Could you check a few things on this model? Use its own coordinates, in mm. A direction names the side the tool comes from. Coordinates: 2 decimals unless noted, no trailing zeros. Order: outer loops, then holes, each group sorted by start corner. A loop starts at its lowest first (then second) coordinate and runs counter-clockwise, first axis right, second up. Notation, with made-up numbers: (-5.75, 28) -> (36.25, 28) arc R16 ccw to (36.25, 42) -> close; hole circle Ø11 at (18.5, 37). An arc over 180 degrees is marked (long way). Use a Markdown table: item, result. Add a question column.
1) If I drill on L1, parallel to Z at x = 1, y = 1; L2, parallel to Z at x = 5, y = 9; L3, parallel to X at y = -0.5, z = -27.5, over which ranges is the centre line in solid material (lowest first)? Write a range as [from, to].
2) Thinking about a two-plate mould opening in X: for faces 1 (the cylindrical face through (-23.31, -13.36, 4.83)), 2 (the flat face through (-15, -3, -3)), 3 (the cylindrical face through (-12.517, -3.694, -1.479)), 4 (the flat face through (12.65, 6.96, 1.48)), which applies, +X half, -X half, draft (parallel to the pull), parting line (faces both ways), or undercut?
3) If we section it at A-A (x = 0): Write out the boundary of the cut face in (y, z), plus the area to 3 significant figures.
4) If we section it at D-D (x = -15): Write out the boundary of the cut face in (y, z), plus the area to 4 significant figures.
5) Will these pins go through, and if not, where does the flat tip stop? pin 1 Ø6 at (x, y) = (17.5, -6) entering from +Z; pin 2 Ø2 at (y, z) = (1, -11) entering from -X; pin 3 Ø1.5 at (x, y) = (-14.5, -3) entering from -Z.
6) If we section it at B-B (z = -27): Write out the boundary of the cut face in (x, y).
7) If we section it at C-C (y = 7): Write out the boundary of the cut face in (x, z), plus the area to 3 significant figures.
8) Which directions (+Z, -Z, +X, -X, +Y, -Y) give clear straight access to the entire face, cutting with the end or side of a thin tool? Please do faces 5 (the flat face through (5, 2, 0)), 6 (the flat face through (-22, -12, 8)), 7 (the flat face through (5, 14, -3)).
```python
from build123d import *

# Parameters (mm, degrees)
BOSS_EXTRUDE1_DEPTH = 3
SKETCH2_R           = 3.5
BOSS_EXTRUDE2_DEPTH = 10
SKETCH3_R           = 2
BOSS_EXTRUDE3_DEPTH = 5
SKETCH4_R           = 2.5
BOSS_EXTRUDE4_DEPTH = 3
CIRPATTERN1_COUNT   = 3
SKETCH5_R           = 3.5
BOSS_EXTRUDE6_DEPTH = 110


with BuildPart() as part:
    # Sketch1 → Boss-Extrude1 (new body)
    with BuildSketch(Plane.XY):
        with BuildLine():
            Line((23.267949192, -11.43375673), (1.732050808, 25.867513459))
            ThreePointArc((1.732050808, 25.867513459), (0, 26.867513459), (-1.732050808, 25.867513459))
            Line((-1.732050808, 25.867513459), (-23.267949192, -11.43375673))
            ThreePointArc((-23.267949192, -11.43375673), (-23.267949192, -13.43375673), (-21.535898385, -14.43375673))
            Line((-21.535898385, -14.43375673), (21.535898385, -14.43375673))
            ThreePointArc((21.535898385, -14.43375673), (23.267949192, -13.43375673), (23.267949192, -11.43375673))
        make_face()
    extrude(amount=BOSS_EXTRUDE1_DEPTH)

    # Sketch2 → Boss-Extrude2 (add)
    with BuildSketch(Plane(origin=(0, 0, 0), x_dir=(-1, 0, 0), z_dir=(0, 0, -1))):
        with Locations(Location((0, 0, 0), (0, 0, 180))):
            Circle(SKETCH2_R)
    extrude(amount=BOSS_EXTRUDE2_DEPTH)

    # Sketch3 → Boss-Extrude3 (add)
    with BuildSketch(Plane.XY.offset(3)):
        with Locations(Location((0, 24.867513459, 0), (0, 0, 150))):
            Circle(SKETCH3_R)
        with Locations(Location((21.535898385, -12.43375673, 0), (0, 0, 270))):
            Circle(SKETCH3_R)
        with Locations(Location((-21.535898385, -12.43375673, 0), (0, 0, 150))):
            Circle(SKETCH3_R)
    extrude(amount=BOSS_EXTRUDE3_DEPTH)

    # Sketch4 → Boss-Extrude4 (add)
    with BuildSketch(Plane(origin=(0, 0, 0), x_dir=(-1, 0, 0), z_dir=(0, 0, -1))):
        with Locations(Location((-10, -11.43375673, 0), (0, 0, 180))):
            Circle(SKETCH4_R)
    boss_extrude4 = extrude(amount=BOSS_EXTRUDE4_DEPTH)

    # CirPattern1: Boss-Extrude4 ×3 about axis
    cirpattern1_axis = Axis((0, 0, 0), (0, 0, 1))
    for i in range(1, CIRPATTERN1_COUNT):
        add(boss_extrude4.rotate(cirpattern1_axis, i * 360 / CIRPATTERN1_COUNT))

    # Sketch5 → Boss-Extrude6 (add)
    with BuildSketch(Plane(origin=(0, 0, -10), x_dir=(-1, 0, 0), z_dir=(0, 0, -1))):
        with Locations(Location((0, 0, 0), (0, 0, 180))):
            Circle(SKETCH5_R)
    extrude(amount=BOSS_EXTRUDE6_DEPTH)


solid = part.part
```
Answer sheet:
| question | item | result |
|---|---|---|
| 1 | L1 | [-120, 3] |
| 1 | L2 | [0, 3] |
| 1 | L3 | [-3.46, 3.46] |
| 2 | face 1 | undercut |
| 2 | face 2 | draft |
| 2 | face 3 | undercut |
| 2 | face 4 | +X half |
| 3 | outline | (-14.43, 0) -> (-3.5, 0) -> (-3.5, -120) -> (3.5, -120) -> (3.5, 0) -> (26.87, 0) -> (26.87, 8) -> (22.87, 8) -> (22.87, 3) -> (-14.43, 3) -> close |
| 3 | area | 984 mm2 |
| 4 | outline | (-14.43, 0) -> (-5.44, 0) -> (-5.44, -3) -> (-0.45, -3) -> (-0.45, 0) -> (2.89, 0) -> (2.89, 3) -> (-14.43, 3) -> close |
| 4 | area | 66.95 mm2 |
| 5 | pin 1 | z = 3 |
| 5 | pin 2 | x = -3.5 |
| 5 | pin 3 | z = -3 |
| 6 | outline | circle Ø7 at (0, 0) |
| 7 | outline | (-12.63, 0) -> (12.63, 0) -> (12.63, 3) -> (-12.63, 3) -> close |
| 7 | area | 75.8 mm2 |
| 8 | face 5 | -Z |
| 8 | face 6 | +Z, +X, -X, +Y, -Y |
| 8 | face 7 | -Z, +X, -X, +Y |
